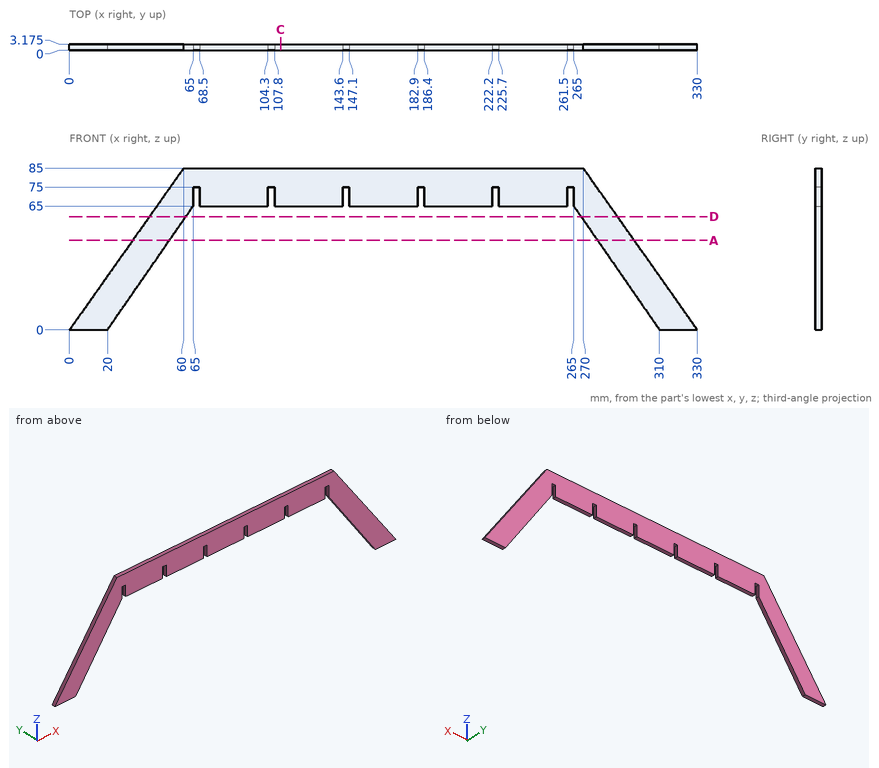
Could you check a few things on this drawing? It's one solid part, dimensions in mm from its lowest x, y, z. Round coordinates to 2 decimals unless told otherwise and drop trailing zeros. Order: outer loops, then holes, each group sorted by start corner. A loop starts at its lowest first (then second) coordinate and runs counter-clockwise, first axis right, second up. Notation, with made-up numbers: M 3,29 L 35,29 A9 ccw 35,46 Z; hole C 50.25,79.25 d8. An arc over 180 degrees is marked long. One line per item, written item: value.
(1) I need wall thicknesses on line 1 along X through (y, z) = (2.1, 11.5); line 2 along Z through (x, y) = (89.5, 0.25); line 3 along X through (y, z) = (1.85, 63.5). Which ranges of each line are inside material? Lowest first, please. Write a range as from..to.
Ans:
line 1: x = 8.12..27.96, 302.04..321.88
line 2: z = 65..85
line 3: x = 44.82..63.96, 266.04..285.18
(2) Imagine slicing it at A-A (z = 47). Write out the boundary of the cut face in (x, y) (3 decimals).
Ans:
outline: M 33.176,0 L 52.538,0 L 52.538,3.175 L 33.176,3.175 Z; M 277.462,0 L 296.824,0 L 296.824,3.175 L 277.462,3.175 Z
(3) Imagine slicing it at D-D (z = 59.5). Write out the boundary of the cut face in (x, y) (3 decimals), and give its area (3 significant figures).
Ans:
outline: M 42,0 L 61.192,0 L 61.192,3.175 L 42,3.175 Z; M 268.808,0 L 288,0 L 288,3.175 L 268.808,3.175 Z
area: 122 mm^2
(4) I'm going to push flat-ended pins straight in: P1, Ø1, axis at y = 1, z = 70.5, coming from the -X side; P2, Ø1, axis at x = 83, y = 1.5, coming from the -Z side; P3, Ø1, axis at x = 67, y = 2, coming from the -Z side. Where does each tip first touch, or does it pass through?
Ans:
P1: stops at x = 49.41
P2: stops at z = 65
P3: stops at z = 75
(5) Imagine slicing it at C-C (x = 111). Write out the boundary of the cut face in (y, z) (3 decimals), and give its area (3 significant figures).
Ans:
outline: M 0,65 L 3.175,65 L 3.175,85 L 0,85 Z
area: 63.5 mm^2
